```python
from build123d import *

# Parameters (mm, degrees)
F1_DEPTH = 30
F3_DEPTH = 10


with BuildPart() as f1:
    # F0 (on Right) → F1 (new body)
    with BuildSketch(Plane.YZ):
        Polygon((0, 15), (0, 0), (30, 0), (30, 30), (10, 30), (10, 15), align=None)
    extrude(amount=F1_DEPTH)

    # F2 (on face) → F3 (cut)
    with BuildSketch(Plane.XZ.offset(-10)):
        Polygon((30, 15), (30, 30), (10, 30), (20, 15), align=None)
    extrude(amount=-F3_DEPTH, mode=Mode.SUBTRACT)


solid = f1.part
```
Check sheet for the modelled part. Datum: model origin and axes. Units: mm. A direction names the side the tool comes from. Coordinates: 2 decimals unless noted, no trailing zeros. Order: outer loops, then holes, each group sorted by start corner. A loop starts at its lowest first (then second) coordinate and runs counter-clockwise, first axis right, second up. Notation, with made-up numbers: M 52,17 L 81,17 A14 cw 81,24 Z; hole C 46,46.5 d1. An arc over 180 degrees is marked long. Write each question's results on one line, items separated by ' | '. Start each with the question number.
1. Cross-section at D-D on x = 12.5. Record the cut outline in (y, z).
2. Go/stop test with flat-tipped pins: P1, Ø10, axis at x = 18.5, y = 11.5, coming from the +Z side; P2, Ø7.5, axis at x = 13, z = 24.5, coming from the -Y side; P3, Ø12, axis at x = 23.5, z = 23, coming from the -Y side. Record where each tip stops, or that it passes through.
3. Cross-section at C-C on y = 17. Record the cut outline in (x, z).
4. Mould release check, pull along X, two halves, no side actions. Record for faces 1 (the face through (8, 10, 23)), 2 (the face through (0, 18, 15)), 3 (the face through (14.93, 14.93, 22.605)): +X half, -X half, draft (parallel to the pull), parting line (faces both ways), or undercut.
5. Access from +Z, -Z, +X, -X, +Y, -Y to the whole of each face (thin tool, end or side, straight path). Record for faces 4 (the face through (18, 8, 15)), 5 (the face through (30, 18, 12)).
6. Material ranges on probe 1 along Z at (x, y) = (11.25, 1.75); probe 2 along Y at (x, z) = (9.5, 26.75); probe 3 along Y at (x, z) = (22.5, 17.75), recorded low to high.
7. Cross-section at B-B on z = 16.5. Record the cut outline in (x, y).
8. Cross-section at A-A on x = 17. Record the cut outline in (y, z), and give its area (3 significant figures).
Checks:
1) outline: M 0,0 L 30,0 L 30,30 L 20,30 L 20,26.25 L 10,26.25 L 10,15 L 0,15 Z
2) P1: stops at z = 24.75 | P2: stops at y = 10 | P3: stops at y = 20
3) outline: M 0,0 L 30,0 L 30,15 L 20,15 L 10,30 L 0,30 Z
4) face 1: draft | face 2: -X half | face 3: +X half
5) face 4: +Z, +X, -Y | face 5: +Z, -Z, +X, +Y, -Y
6) probe 1: z = 0 to 15 | probe 2: y = 10 to 30 | probe 3: y = 20 to 30
7) outline: M 0,10 L 19,10 L 19,20 L 30,20 L 30,30 L 0,30 Z
8) outline: M 0,0 L 30,0 L 30,30 L 20,30 L 20,19.5 L 10,19.5 L 10,15 L 0,15 Z | area: 645 mm²
